Geometry: final body of the model. Coordinates: model frame, mm. Face numbers are marked on the shaded views. Round coordinates to 2 decimals unless told otherwise and drop trailing zeros. Loops run counter-clockwise (first coordinate to the right, second up) from the corner with the lowest first, then second, coordinate; pieces in that order, holes last. Notation, with made-up numbers: (53.25, 83) - (59.25, 83) arc R34 ccw to (59.25, 114) - close; hole circle Ø7 at (-4.75, -5). An arc over 180 degrees is marked (long way). Return JSON: item names as keys, results as strings. Group by question number.
1. Section D-D on z = -9. Return loops of the section in (x, y).
2. Draft query along Z for the marked faces 1, 2 and 3. Return one class per face: +Z half, -Z half, draft (parallel to the pull), parting line (faces both ways), or undercut.
3. Material intervals for probe 1 along X at (y, z) = (1.1, 0); probe 2 along X at (y, z) = (0.5, 9); probe 3 along Z at (x, y) = (-1.75, 1), sorted ascending.
4. Section B-B on z = 0. Return loops of the section in (x, y), and give its area (3 significant figures).
5. Section C-C on y = 1.65. Return loops of the section in (x, z).
6. Section A-A on x = 9. Return loops of the section in (y, z), and give its area (3 significant figures).
from build123d import *

# Parameters (mm, degrees)
SKETCH1_R           = 1.1
SKETCH1_R_2         = 6.15
BOSS_EXTRUDE1_DEPTH = 2


with BuildPart() as part:
    # Sketch1 → Boss-Extrude1 (new body)
    with BuildSketch(Plane(origin=(0, 0, 0), x_dir=(1, 0, 0), z_dir=(0, 1, 0))):
        with BuildLine():
            ThreePointArc((-2.717716562, -8.579861111), (0, -11.75), (2.717716562, -8.579861111))
            ThreePointArc((2.717716562, -8.579861111), (6.363961031, -6.363961031), (8.579861111, -2.717716562))
            ThreePointArc((8.579861111, -2.717716562), (11.75, 0), (8.579861111, 2.717716562))
            ThreePointArc((8.579861111, 2.717716562), (6.363961031, 6.363961031), (2.717716562, 8.579861111))
            ThreePointArc((2.717716562, 8.579861111), (0, 11.75), (-2.717716562, 8.579861111))
            ThreePointArc((-2.717716562, 8.579861111), (-6.363961031, 6.363961031), (-8.579861111, 2.717716562))
            ThreePointArc((-8.579861111, 2.717716562), (-11.75, 0), (-8.579861111, -2.717716562))
            ThreePointArc((-8.579861111, -2.717716562), (-6.363961031, -6.363961031), (-2.717716562, -8.579861111))
        make_face()
        with Locations(Location((0, -9, 0), (0, 0, 270))):
            Circle(SKETCH1_R, mode=Mode.SUBTRACT)
        with Locations(Location((-9, 0, 0), (0, 0, 270))):
            Circle(SKETCH1_R, mode=Mode.SUBTRACT)
        with Locations(Location((0, 0, 0), (0, 0, 270))):
            Circle(SKETCH1_R_2, mode=Mode.SUBTRACT)
        with Locations(Location((9, 0, 0), (0, 0, 270))):
            Circle(SKETCH1_R, mode=Mode.SUBTRACT)
        with Locations(Location((0, 9, 0), (0, 0, 270))):
            Circle(SKETCH1_R, mode=Mode.SUBTRACT)
    extrude(amount=BOSS_EXTRUDE1_DEPTH)


solid = part.part
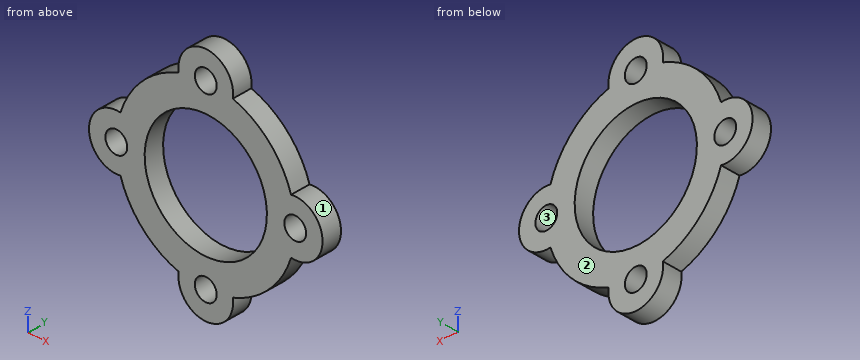
Taken from the geometry:
{
 "1": {"outline": "(-2.75, 0) - (-1.1, 0) - (-1.1, 2) - (-2.75, 2) - close; (1.1, 0) - (2.75, 0) - (2.75, 2) - (1.1, 2) - close"},
 "2": {"face 1": "parting line", "face 2": "draft", "face 3": "undercut"},
 "3": {"probe 1": "-11.75 to -10.1, -7.9 to -6.15, 6.15 to 7.9, 10.1 to 11.75", "probe 2": "-2.75 to -1.1, 1.1 to 2.75", "probe 3": "-11.12 to -5.9, 5.9 to 11.12"},
 "4": {"outline": "(-11.75, 0) - (-10.1, 0) - (-10.1, 2) - (-11.75, 2) - close; (-7.9, 0) - (-6.15, 0) - (-6.15, 2) - (-7.9, 2) - close; (6.15, 0) - (7.9, 0) - (7.9, 2) - (6.15, 2) - close; (10.1, 0) - (11.75, 0) - (11.75, 2) - (10.1, 2) - close", "area": "13.6 mm2"},
 "5": {"outline": "(-8.58, -2.72) arc R9 ccw to (-2.72, -8.58) arc R2.75 ccw (long way) to (2.72, -8.58) arc R9 ccw to (8.58, -2.72) arc R2.75 ccw (long way) to (8.58, 2.72) arc R9 ccw to (2.72, 8.58) arc R2.75 ccw (long way) to (-2.72, 8.58) arc R9 ccw to (-8.58, 2.72) arc R2.75 ccw (long way) to start; hole circle Ø2.2 at (-9, 0); hole circle Ø12.3 at (0, 0); hole circle Ø2.2 at (0, -9); hole circle Ø2.2 at (0, 9); hole circle Ø2.2 at (9, 0)"},
 "6": {"outline": "(0, -2.75) - (2, -2.75) - (2, -1.1) - (0, -1.1) - close; (0, 1.1) - (2, 1.1) - (2, 2.75) - (0, 2.75) - close", "area": "6.60 mm2"}
}
